Source: CAD feature listing. Evaluate the final solid. Frame: model axes, mm. Round coordinates to 2 decimals unless told otherwise and drop trailing zeros. Order: outer loops, then holes, each group sorted by start corner. A loop starts at its lowest first (then second) coordinate and runs counter-clockwise, first axis right, second up. Notation, with made-up numbers: (-27, -5.5) - (-6, -5.5) arc R16 ccw to (-6, 24.5) - close; hole circle Ø10 at (44, 60). An arc over 180 degrees is marked (long way). Use one line per item in the form item = value. Start each with the question number.
Q1. Ray query, line 1 (Z direction, x = 2.5, y = 4.25); line 2 (Y direction, x = 2.5, z = 3.5); line 3 (Y direction, x = 9.5, z = -3.75). Return the intervals inside material, ascending. Write a range as [from, to].
Q2. Cut plane C-C, the plane y = 10.5. Return the cut outline in (x, z).
Q3. Cut plane A-A, the plane y = 4.5. Give the number of separate pieces and of enclosed holes in the cut face, and give its area (3 significant figures).
Q4. Cut plane B-B, the plane x = 8.25. Return the cut outline in (y, z).
Q5. Pin query (flat end, axial travel): pin 1 Ø1.5 at (x, z) = (3.5, 1) entering from +Y; pin 2 Ø3 at (x, z) = (4, -0.5) entering from -Y; pin 3 Ø5 at (x, z) = (7, -5) entering from +Y. Return the tip coordinate at first contact, or that it passes through.
from build123d import *

# Parameters (mm, degrees)
BOSS_EXTRUDE1_DEPTH                               = 6.35
CSK_FOR_4_FLAT_HEAD_MACHINE_SCREW_100_D           = 3.2639
CSK_FOR_4_FLAT_HEAD_MACHINE_SCREW_100_CSINK_D     = 5.715
CSK_FOR_4_FLAT_HEAD_MACHINE_SCREW_100_CSINK_ANGLE = 100


with BuildPart() as part:
    # Sketch1 → Boss-Extrude1 (new body, symmetric)
    with BuildSketch(Plane.XY):
        Polygon((0, 11.596551211), (11.596551211, 0), (5.656854249, 0), (0, 5.656854249), align=None)
    extrude(amount=BOSS_EXTRUDE1_DEPTH, both=True)

    # CSK for #4 Flat Head Machine Screw (100)1 (through all)
    with Locations(Plane(origin=(2.828427125, 2.828427125, 0), x_dir=(0, 0, 1), z_dir=(-0.707106781, -0.707106781, 0))):
        with Locations((-3.175, -0.224693873), (3.175, -0.224693873)):
            CounterSinkHole(CSK_FOR_4_FLAT_HEAD_MACHINE_SCREW_100_D / 2, CSK_FOR_4_FLAT_HEAD_MACHINE_SCREW_100_CSINK_D / 2, counter_sink_angle=CSK_FOR_4_FLAT_HEAD_MACHINE_SCREW_100_CSINK_ANGLE)


solid = part.part
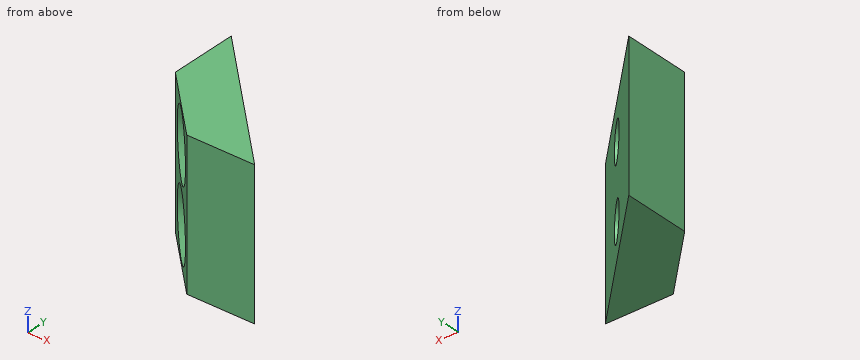
Completed:
q1.line_1 = [-6.35, -4.44], [-1.91, 1.91], [4.44, 6.35]
q1.line_2 = [4.54, 9.1]
q1.line_3 = [0, 2.1]
q2.outline = (0, -6.35) - (1.1, -6.35) - (1.1, 6.35) - (0, 6.35) - close
q3.separate_pieces = 3
q3.enclosed_holes = 0
q3.area = 47.0 mm2
q4.outline = (0, -6.35) - (3.35, -6.35) - (3.35, 6.35) - (0, 6.35) - close
q5.pin_1 = 8.85
q5.pin_2 = 0.16
q5.pin_3 = 7.1
